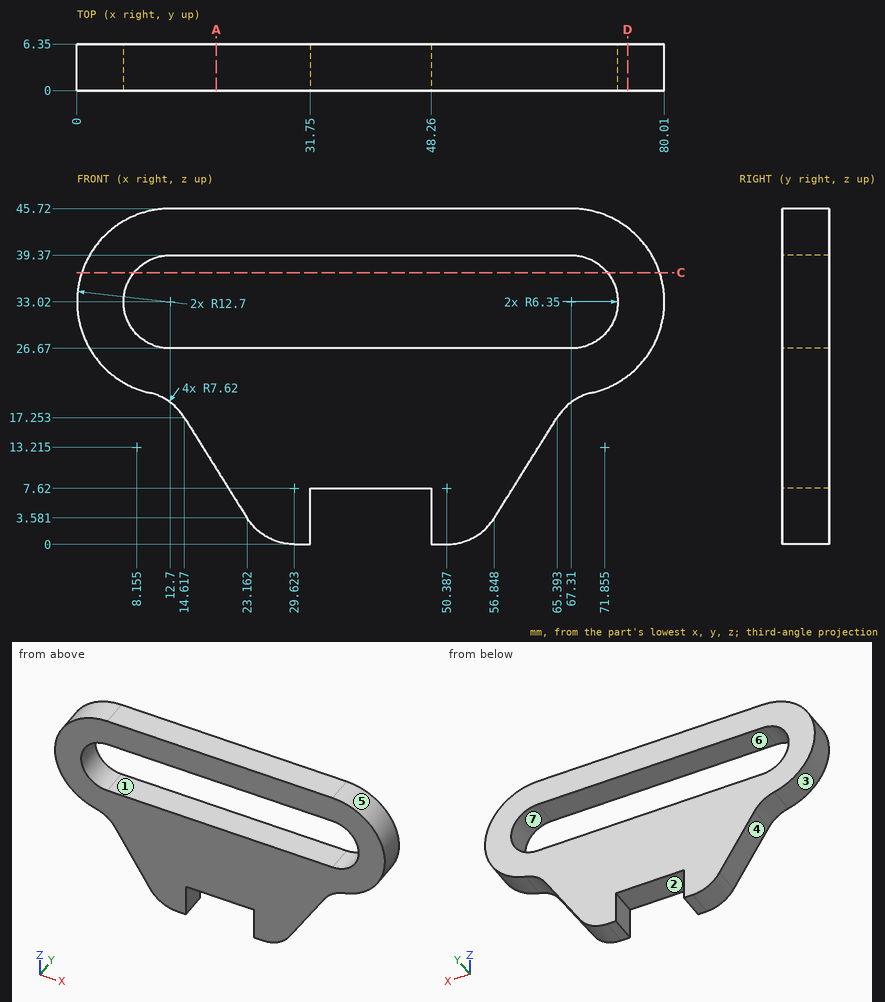
Could you check a few things on this drawing? It's one solid part, dimensions in mm from its lowest x, y, z. A direction names the side the tool comes from. Give positions to 0.01 mm unless a question says otherwise; leave off trailing zeros. Order: outer loops, then holes, each group sorted by start corner. A loop starts at its lowest first (then second) coordinate and runs counter-clockwise, first axis right, second up.
1. Suppose I cut it at C-C (z = 37). Write out the boundary of the cut face in (x, y).
Answers below:
outline: (0.64, 0) - (7.75, 0) - (7.75, 6.35) - (0.64, 6.35) - close; (72.26, 0) - (79.37, 0) - (79.37, 6.35) - (72.26, 6.35) - close
2. Which directions (+Z, -Z, +X, -X, +Y, -Y) give clear straight access to the entire face, cutting with the end or side of a thin tool? Please do the marked faces 1, 2 and 3.
Answers below:
face 1: +Y, -Y
face 2: -Z, +Y, -Y
face 3: -X, +Y, -Y
3. Suppose I cut it at D-D (x = 75). Write out the boundary of the cut face in (y, z).
Answers below:
outline: (0, 22.91) - (6.35, 22.91) - (6.35, 43.13) - (0, 43.13) - close
4. Suppose I cut it at A-A (x = 19). Write out the boundary of the cut face in (y, z), plus the area to 3 significant figures.
Answers below:
outline: (0, 10.24) - (6.35, 10.24) - (6.35, 26.67) - (0, 26.67) - close; (0, 39.37) - (6.35, 39.37) - (6.35, 45.72) - (0, 45.72) - close
area: 145 mm2
5. I need wall thicknesses on L1, parallel to Z at x = 50, y = 5.75; L2, parallel to Z at x = 46, y = 0.5; L3, parallel to X at y = 2, z = 4.5. Which ranges of each line are inside material? Lowest first, please.
Answers below:
L1: z = 0 to 26.67, 39.37 to 45.72
L2: z = 7.62 to 26.67, 39.37 to 45.72
L3: x = 22.59 to 31.75, 48.26 to 57.42
6. For pin 1 (1.9 mm diameter, centred on y = 3.5, z = 3.5, fed in from -X), with a flat end and sliding along its axis, tell me the tip position at first contact or that it passes through.
Answers below:
pin 1: stops at x = 22.62
7. Thinking about a two-plate mould opening in Z: for the marked faces 4, 5, 6 and 7, which applies, +Z half, -Z half, draft (parallel to the pull), parting line (faces both ways), or undercut?
Answers below:
face 4: -Z half
face 5: parting line
face 6: undercut
face 7: undercut
